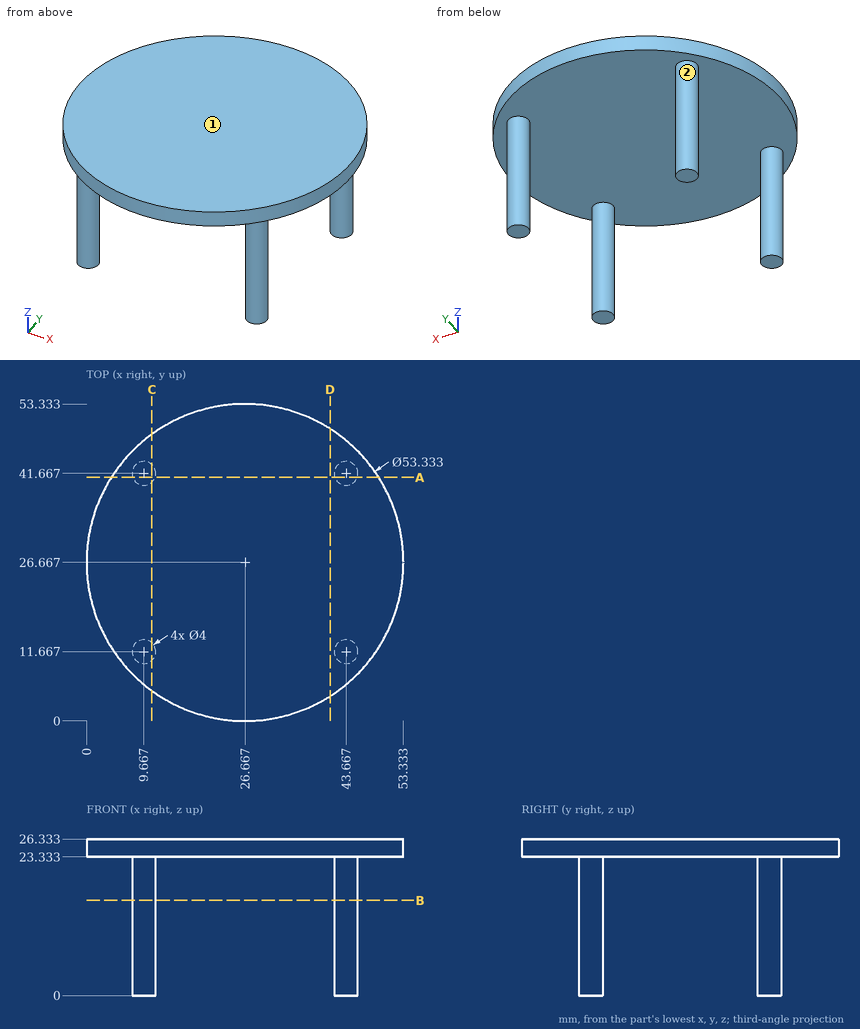
Geometry: see drawing. Coordinates: mm, zero at the bounding-box minimum. Round coordinates to 2 decimals unless told otherwise and drop trailing zeros. Order: outer loops, then holes, each group sorted by start corner. A loop starts at its lowest first (then second) coordinate and runs counter-clockwise, first axis right, second up. Notation, with made-up numbers: (83, 42) -> (89, 42) arc R9 cw to (89, 48) -> close; hole circle Ø4 at (50.5, 71.5). An arc over 180 degrees is marked (long way). Write each question's results on one line, items separated by ' | '.
Q1. Section query C-C (x = 11). Output: boundary loops of the cut face in (y, z).
Response values:
outline: (5.09, 23.33) -> (10.18, 23.33) -> (10.18, 0) -> (13.16, 0) -> (13.16, 23.33) -> (40.18, 23.33) -> (40.18, 0) -> (43.16, 0) -> (43.16, 23.33) -> (48.25, 23.33) -> (48.25, 26.33) -> (5.09, 26.33) -> close
Q2. Section query D-D (x = 41). Output: boundary loops of the cut face in (y, z).
Response values:
outline: (4.18, 23.33) -> (49.15, 23.33) -> (49.15, 26.33) -> (4.18, 26.33) -> close
Q3. Section query A-A (y = 41). Output: boundary loops of the cut face in (x, z), and give its area (3 significant figures).
Response values:
outline: (4.18, 23.33) -> (7.78, 23.33) -> (7.78, 0) -> (11.55, 0) -> (11.55, 23.33) -> (41.78, 23.33) -> (41.78, 0) -> (45.55, 0) -> (45.55, 23.33) -> (49.15, 23.33) -> (49.15, 26.33) -> (4.18, 26.33) -> close | area: 311 mm²
Q4. Pin query (flat end, axial travel): pin 1 Ø1 at (x, y) = (36, 37) entering from -Z; pin 2 Ø10 at (x, z) = (41, 4) entering from +Y; pin 3 Ø1.5 at (x, z) = (11, 4) entering from -Y. Return the tip coordinate at first contact, or that it passes through.
Response values:
pin 1: z = 23.33 | pin 2: y = 43.67 | pin 3: y = 9.75
Q5. Ray query, line 1 along Z through (x, y) = (16, 25); line 2 along X through (y, z) = (41.5, 9.5); line 3 along Y through (x, z) = (42.5, 8.25). Return the intervals inside material, ascending.
Response values:
line 1: 23.33 to 26.33 | line 2: 7.67 to 11.66, 41.67 to 45.66 | line 3: 10.04 to 13.29, 40.04 to 43.29
Q6. Section query B-B (z = 16). Output: boundary loops of the cut face in (x, y).
Response values:
outline: circle Ø4 at (9.67, 11.67); circle Ø4 at (9.67, 41.67); circle Ø4 at (43.67, 11.67); circle Ø4 at (43.67, 41.67)
Q7. Pull-direction query (X, two-part tool) for the marked faces 1 and 2; classes: released by +X, released by -X, zero draft, split by the parting line, or undercut.
Response values:
face 1: zero draft | face 2: undercut
